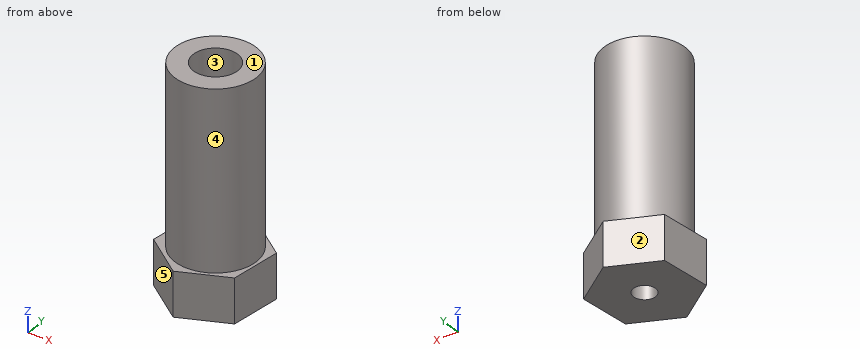
from build123d import *

# Parameters (mm, degrees)
BOSS_EXTRUDE1_DEPTH = 6
SKETCH3_R           = 5.5
BOSS_EXTRUDE2_DEPTH = 24
SKETCH4_R           = 1.5
CUT_EXTRUDE1_DEPTH  = 6
SKETCH5_R           = 3
CUT_EXTRUDE2_DEPTH  = 24


with BuildPart() as part:
    # Sketch1 → Boss-Extrude1 (new body)
    with BuildSketch(Plane.XY):
        Polygon((0.950381036, -2.263552428), (1.849306406, 4.606086076), (-3.650512368, 8.819397535), (-10.049256513, 6.163070489), (-10.948181883, -0.706568015), (-5.448363108, -4.919879474), align=None)
    extrude(amount=BOSS_EXTRUDE1_DEPTH)

    # Sketch3 → Boss-Extrude2 (add)
    with BuildSketch(Plane.XY.offset(6)):
        with Locations((-4.462077205, 1.925315909)):
            Circle(SKETCH3_R)
    extrude(amount=BOSS_EXTRUDE2_DEPTH)

    # Sketch4 → Cut-Extrude1 (cut)
    with BuildSketch(Plane(origin=(0, 0, 0), x_dir=(-1, 0, 0), z_dir=(0, 0, -1))):
        with Locations((4.462077205, 1.925315909)):
            Circle(SKETCH4_R)
    extrude(amount=-CUT_EXTRUDE1_DEPTH, mode=Mode.SUBTRACT)

    # Sketch5 → Cut-Extrude2 (cut)
    with BuildSketch(Plane.XY.offset(30)):
        with Locations((-4.462077205, 1.925315909)):
            Circle(SKETCH5_R)
    extrude(amount=-CUT_EXTRUDE2_DEPTH, mode=Mode.SUBTRACT)


solid = part.part
Verification items for the finished model (mm, model axes). Face numbers are marked on the shaded views. A direction names the side the tool comes from. Coordinates: 2 decimals unless noted, no trailing zeros. Write each loop counter-clockwise with the first axis right and the second up, starting at its lowest first coordinate (ties: lowest second). Pieces come first, ordered by that corner, then holes. Notation, with made-up numbers: M 61.25,-7.75 L 98.25,-7.75 A21 ccw 98.25,26.25 Z; hole C 37,-31 d4. An arc over 180 degrees is marked long. Use a Markdown table: item, result.
Q1. Set-up check for the marked faces 4 and 5: record each of +Z, -Z, +X, -X, +Y, -Y from which the full face is reachable in a straight line by a thin tool's end or side.
Reply:
| item | result |
|---|---|
| face 4 | +Z |
| face 5 | +Z, -Z, -X, -Y |
Q2. Sectioned sample at C-C, the plane y = 3. Record the boundary of the cut face in (x, z), plus the area to 3 significant figures.
Reply:
| item | result |
|---|---|
| outline | M -10.46,0 L -5.51,0 L -5.51,6 L -7.26,6 L -7.26,30 L -9.86,30 L -9.86,6 L -10.46,6 Z; M -3.42,0 L 1.64,0 L 1.64,6 L 0.93,6 L 0.93,30 L -1.66,30 L -1.66,6 L -3.42,6 Z |
| area | 185 mm² |
Q3. Draft check along X on the marked faces 1, 2 and 3. Enter one of: +X half, -X half, draft (parallel to the pull), parting line (faces both ways), or undercut.
Reply:
| item | result |
|---|---|
| face 1 | draft |
| face 2 | -X half |
| face 3 | undercut |
Q4. Go/stop test with flat-tipped pins: P1, Ø3.5, axis at x = -4.46, y = 1.93, coming from the +Z side; P2, Ø1.5, axis at y = 3.5, z = 25.5, coming from the +X side; P3, Ø1, axis at x = -4, z = 26.5, coming from the -Y side. Record where each tip stops, or that it passes through.
Reply:
| item | result |
|---|---|
| P1 | stops at z = 6 |
| P2 | stops at x = 0.98 |
| P3 | stops at y = -3.57 |
Q5. Sectioned sample at B-B, the plane x = -4.75. Record the boundary of the cut face in (y, z), plus the area to 3 significant figures.
Reply:
| item | result |
|---|---|
| outline | M -4.63,0 L 0.45,0 L 0.45,6 L -1.06,6 L -1.06,30 L -3.57,30 L -3.57,6 L -4.63,6 Z; M 3.4,0 L 8.36,0 L 8.36,6 L 7.42,6 L 7.42,30 L 4.91,30 L 4.91,6 L 3.4,6 Z |
| area | 181 mm² |
Q6. Sectioned sample at D-D, the plane x = -7. Record the boundary of the cut face in (y, z), plus the area to 3 significant figures.
Reply:
| item | result |
|---|---|
| outline | M -3.73,0 L 7.43,0 L 7.43,6 L 6.8,6 L 6.8,30 L 3.52,30 L 3.52,6 L 0.33,6 L 0.33,30 L -2.95,30 L -2.95,6 L -3.73,6 Z |
| area | 224 mm² |
Q7. Sectioned sample at A-A, the plane z = 2.5. Record the boundary of the cut face in (x, y).
Reply:
| item | result |
|---|---|
| outline | M -10.95,-0.71 L -5.45,-4.92 L 0.95,-2.26 L 1.85,4.61 L -3.65,8.82 L -10.05,6.16 Z; hole C -4.46,1.93 d3 |
Q8. Thickness scan on line 1 (X direction, y = 1.75, z = 25.75); line 2 (Z direction, x = -3.25, y = 0.75); line 3 (X direction, y = -0.75, z = 7.25). Record the ranges inside material, lowest first.
Reply:
| item | result |
|---|---|
| line 1 | x = -9.96 to -7.46, -1.47 to 1.04 |
| line 2 | z = 0 to 6 |
| line 3 | x = -9.27 to -5.82, -3.1 to 0.34 |
